from build123d import *

# Parameters (mm, degrees)
F0_R     = 19.05
F1_DEPTH = 152.4
F2_W     = 88.9
F2_H     = 63.5
F3_DEPTH = 88.9
F4_R     = 19.05
F5_R     = 5.08
F6_DEPTH = 152.4
F8_DEPTH = 241.301
F9_R     = 5.08
F10_R    = 5.08


with BuildPart() as f1:
    # F0 (on Front) → F1 (new body)
    with BuildSketch(Plane.XZ):
        Circle(F0_R)
    extrude(amount=F1_DEPTH)

    # F2 (on face) → F3 (join)
    with BuildSketch(Plane(origin=(0, 0, 0), x_dir=(-1, 0, 0), z_dir=(0, 1, 0))):
        Rectangle(F2_W, F2_H)
    extrude(amount=F3_DEPTH)

    # F4
    f4_edges = [f1.edges().sort_by_distance(p)[0] for p in [
        (44.45, 44.45, 31.75),
        (-44.45, 44.45, 31.75),
        (-44.45, 44.45, -31.75),
        (44.45, 44.45, -31.75),
    ]]
    fillet(f4_edges, radius=F4_R)

    # F5 (on face) → F6 (cut, through all)
    with BuildSketch(Plane.XZ.offset(152.4)):
        Circle(F5_R)
        with BuildLine():
            ThreePointArc((3.7909021354, 18.669), (0, 19.05), (-3.7909021354, 18.669))
            ThreePointArc((-3.7909021354, 18.669), (0, 15.24), (3.7909021354, 18.669))
        make_face()
        with BuildLine():
            ThreePointArc((-18.0632793309, -6.0514824475), (-16.4977839421, -9.525), (-14.2723771956, -12.6175175525))
            ThreePointArc((-14.2723771956, -12.6175175525), (-13.1982271537, -7.62), (-18.0632793309, -6.0514824475))
        make_face()
        with BuildLine():
            ThreePointArc((14.2723771956, -12.6175175525), (16.4977839421, -9.525), (18.0632793309, -6.0514824475))
            ThreePointArc((18.0632793309, -6.0514824475), (13.1982271537, -7.62), (14.2723771956, -12.6175175525))
        make_face()
    extrude(amount=-F6_DEPTH, mode=Mode.SUBTRACT)

    # F7 (on face) → F8 (cut, through all)
    with BuildSketch(Plane(origin=(0, 88.9, 0), x_dir=(-1, 0, 0), z_dir=(0, 1, 0))):
        Polygon((9.525, 31.75), (0, 31.75), (-9.525, 31.75), (-12.7, 28.575), (-9.525, 25.4), (0, 25.4), (9.525, 25.4), (12.7, 28.575), align=None)
    extrude(amount=-F8_DEPTH, mode=Mode.SUBTRACT)

    # F9
    f9_edges = [f1.edges().sort_by_distance(p)[0] for p in [
        (3.790902, -76.2, 18.669),
        (-3.790902, -76.2, 18.669),
        (-14.272377, -76.2, -12.617518),
        (-18.063279, -76.2, -6.051482),
        (18.063279, -76.2, -6.051482),
        (14.272377, -76.2, -12.617518),
    ]]
    fillet(f9_edges, radius=F9_R)

    # F10
    f10_edges = [f1.edges().sort_by_distance(p)[0] for p in [
        (44.45, 0, 0),
        (44.45, 88.9, 0),
    ]]
    fillet(f10_edges, radius=F10_R)


solid = f1.part
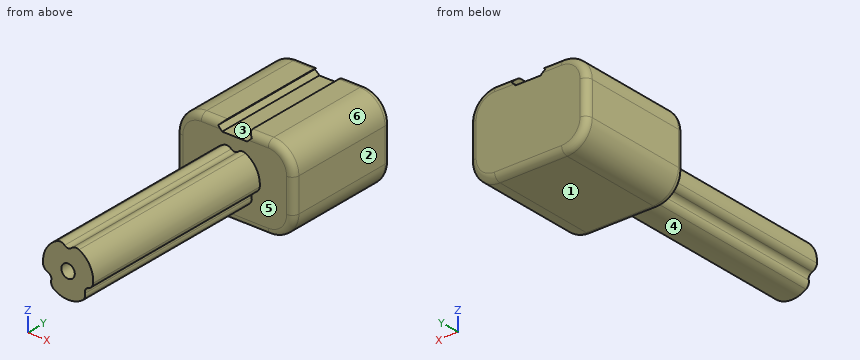
Build history of the part. All positions in model axes, mm. Face numbers are marked on the shaded views. A direction names the side the tool comes from. Coordinates: 2 decimals unless noted, no trailing zeros. Write each loop counter-clockwise with the first axis right and the second up, starting at its lowest first coordinate (ties: lowest second). Pieces come first, ordered by that corner, then holes. Notation, with made-up numbers: (55.5, 66.5) -> (98.5, 66.5) arc R32 ccw to (98.5, 101.5) -> close; hole circle Ø4 at (-36, -5.75). An arc over 180 degrees is marked (long way). Use CSV: the item, a comma, the result in double quotes. Start each with the question number.
Q1. Drill centre lines: probe 1 along Y at (x, z) = (-3, 4); probe 2 along X at (y, z) = (-131.5, -4); probe 3 along X at (y, z) = (-125, -2.5). Where is each one in solid material? Low to high.
Q2. 3-axis set-ups, long thin cutter, end or side, ignore diameter. For the marked faces 5 and 6: which of +Z, -Z, +X, -X, +Y, -Y reach the whole face in a straight line?
Q3. Cut at B-B, the plane z = 8.5. List the corners of the cut face in (x, y).
Q4. Flat gauge pins, fed straight in: pin 1 Ø1.5 at (x, y) = (-10.5, -105) entering from +Z; pin 2 Ø1 at (y, z) = (31.5, -19.5) entering from -X; pin 3 Ø5 at (y, z) = (-66, -9.5) entering from -X. Where does each tip first touch, or does it go through?
Q5. Pull direction X, two halves, no side cores. Call the marked faces 1, 2, 3 and 4: released by +X, released by -X, zero draft, split by the parting line, or undercut.
Q6. Cut at A-A, the plane x = 0. List the corners of the cut face in (y, z).
Checked values:
1,probe 1,"y = 0 to 88.9"
1,probe 2,"x = -18.04 to -3.13, 3.13 to 18.04"
1,probe 3,"x = -18.79 to -4.42, 4.42 to 18.79"
2,face 5,"-Y"
2,face 6,"+Z, +X, +Y, -Y"
3,outline,"(-44.45, 5.08) arc R5.08 ccw to (-39.37, 0) -> (-17.05, 0) -> (-17.05, -152.4) -> (17.05, -152.4) -> (17.05, 0) -> (39.37, 0) arc R5.08 ccw to (44.45, 5.08) -> (44.45, 83.82) arc R5.08 ccw to (39.37, 88.9) -> (-39.37, 88.9) arc R5.08 ccw to (-44.45, 83.82) -> close"
4,pin 1,"stops at z = 16.37"
4,pin 2,"stops at x = -43.38"
4,pin 3,"stops at x = -13.64"
5,face 1,"zero draft"
5,face 2,"released by +X"
5,face 3,"undercut"
5,face 4,"split by the parting line"
6,outline,"(-152.4, -19.05) -> (0, -19.05) -> (0, -26.67) arc R5.08 ccw to (5.08, -31.75) -> (83.82, -31.75) arc R5.08 ccw to (88.9, -26.67) -> (88.9, 25.4) -> (0, 25.4) -> (0, 15.24) -> (-152.4, 15.24) -> (-152.4, 5.08) -> (0, 5.08) -> (0, -5.08) -> (-152.4, -5.08) -> close"
